Source: CAD feature listing. Evaluate the final solid. Frame: model axes, mm. Face numbers are marked on the shaded views. A direction names the side the tool comes from. Give positions to 0.01 mm unless a question says otherwise; leave off trailing zeros. Order: outer loops, then holes, each group sorted by start corner. A loop starts at its lowest first (then second) coordinate and runs counter-clockwise, first axis right, second up. Notation, with made-up numbers: (68.25, 3.25) - (111.25, 3.25) arc R15 ccw to (111.25, 32.25) - close; hole circle Ø2 at (50.25, -12). An arc over 180 degrees is marked (long way). Answer as CSV lines item,"result".
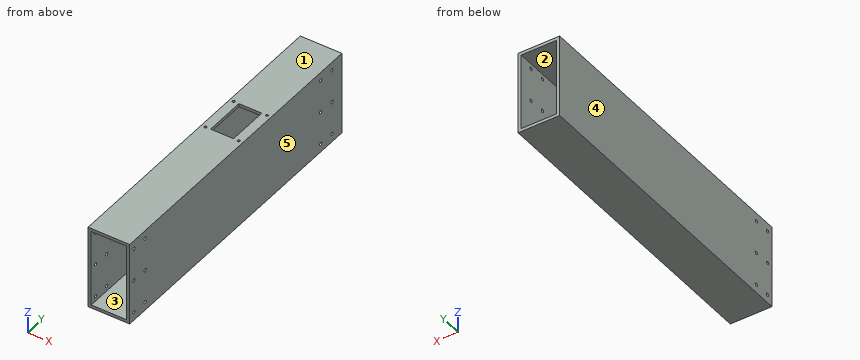
```python
from build123d import *

# Parameters (mm, degrees)
SKETCH1_W                        = 40
SKETCH1_H                        = 80
SKETCH1_W_2                      = 34
SKETCH1_H_2                      = 74
BOSS_EXTRUDE1_DEPTH              = 300
CUT_EXTRUDE1_REACH               = 315.05
SKETCH2_W                        = 22
SKETCH2_H                        = 40
TAP_DRILL_FOR_M3_TAP1_D          = 2.5
TAP_DRILL_FOR_M3_TAP1_DEPTH      = 3
TAP_DRILL_FOR_M3_HELICOIL1_D     = 3.15
TAP_DRILL_FOR_M3_HELICOIL2_D     = 3.15
TAP_DRILL_FOR_M3_HELICOIL2_DEPTH = 3


with BuildPart() as part:
    # Sketch1 → Boss-Extrude1 (new body)
    with BuildSketch(Plane(origin=(0, 0, 0), x_dir=(1, 0, 0), z_dir=(0, 1, 0))):
        with Locations((20, 40)):
            Rectangle(SKETCH1_W, SKETCH1_H)
        with Locations((20, 40)):
            Rectangle(SKETCH1_W_2, SKETCH1_H_2, mode=Mode.SUBTRACT)
    extrude(amount=BOSS_EXTRUDE1_DEPTH)

    # Sketch2 → Cut-Extrude1 (cut, up to next)
    with BuildSketch(Plane.XY, mode=Mode.PRIVATE) as cut_extrude1_sk1:
        with Locations((20, 180)):
            Rectangle(SKETCH2_W, SKETCH2_H)
    cut_extrude1_tool1 = extrude(cut_extrude1_sk1.sketch, amount=-CUT_EXTRUDE1_REACH, mode=Mode.PRIVATE) & part.part
    add(cut_extrude1_tool1.solids().sort_by_distance((20, 180, 0))[0], mode=Mode.SUBTRACT)

    # Tap Drill for M3 Tap1
    with Locations(Plane.XY):
        with Locations((4, 200), (36, 200), (36, 160), (4, 160)):
            Hole(TAP_DRILL_FOR_M3_TAP1_D / 2, depth=TAP_DRILL_FOR_M3_TAP1_DEPTH)

    # Tap Drill for M3 Helicoil1 (through all)
    with Locations(Plane.ZY):
        with Locations((-8, 6), (-40, 6), (-72, 6), (-40, 22), (-72, 22), (-8, 22)):
            Hole(TAP_DRILL_FOR_M3_HELICOIL1_D / 2)

    # Tap Drill for M3 Helicoil2
    with Locations(Plane(origin=(40, 0, 0), x_dir=(0, 0, -1), z_dir=(1, 0, 0))):
        with Locations((72, 286), (72, 270), (40, 286), (40, 270), (8, 286), (8, 270)):
            Hole(TAP_DRILL_FOR_M3_HELICOIL2_D / 2, depth=TAP_DRILL_FOR_M3_HELICOIL2_DEPTH)


solid = part.part
```
(1) Ray query, line 1 (Y direction, x = 2.3, z = -72) (3 decimals); line 2 (Y direction, x = 39.25, z = -72) (3 decimals); line 3 (Y direction, x = 36, z = -2.1). Return the intervals inside material, ascending. Write a range as from..to.
Completed:
line 1,"0..4.425, 7.575..20.425, 23.575..300"
line 2,"0..4.425, 7.575..20.425, 23.575..268.425, 271.575..284.425, 287.575..300"
line 3,"0..158.75, 161.25..198.75, 201.25..300"
(2) Cut plane B-B (x = 22.5). Return loops of the section in (y, z).
Completed:
outline,"(0, -80) - (300, -80) - (300, -77) - (0, -77) - close; (0, -3) - (160, -3) - (160, 0) - (0, 0) - close; (200, -3) - (300, -3) - (300, 0) - (200, 0) - close"
(3) Cut plane C-C (y = 173). Return loops of the section in (x, z), then the cut area to 3 significant figures.
Completed:
outline,"(0, -80) - (40, -80) - (40, 0) - (31, 0) - (31, -3) - (37, -3) - (37, -77) - (3, -77) - (3, -3) - (9, -3) - (9, 0) - (0, 0) - close"
area,"618 mm²"
(4) Cut plane A-A (z = -22). Return loops of the section in (x, y), then the cut area to 3 significant figures.
Completed:
outline,"(0, 0) - (3, 0) - (3, 300) - (0, 300) - close; (37, 0) - (40, 0) - (40, 300) - (37, 300) - close"
area,"1,800 mm²"
(5) Mould query, pull axis X, two halves, no side actions, for the marked faces 3, 4 and 5. Classes: released by +X, released by -X, zero draft, split by the parting line, or undercut.
Completed:
face 3,"undercut"
face 4,"released by -X"
face 5,"released by +X"
(6) Contact query for a flat-ended pin moving along its axis: pin 1 (2.5 mm diameter, centred on y = 286, z = -40, fed in from +X). Output: stop coordinate, or through.
Completed:
pin 1,"x = 3"
(7) Access query for the marked faces 1 and 2. Directions: +Z, -Z, +X, -X, +Y, -Y. A direction counts if a zero-diameter tool reaches every point of the face in a straight line with its end or side. Return the directions, or none.
Completed:
face 1,"+Z, +X, -X, +Y, -Y"
face 2,"+Y, -Y"
